Here's the drawing with two shaded views (mm, measured from the low corner). I have some questions. A direction names the side the tool comes from. Round coordinates to 2 decimals unless told otherwise and drop trailing zeros. Loops run counter-clockwise (first coordinate to the right, second up) from the corner with the lowest first, then second, coordinate; pieces in that order, holes last. Notation, with made-up numbers: M 89.25,65 L 141.25,65 A18 ccw 141.25,82 Z; hole C -29,81.25 d3. An arc over 180 degrees is marked long. Answer as CSV lines item,"result".
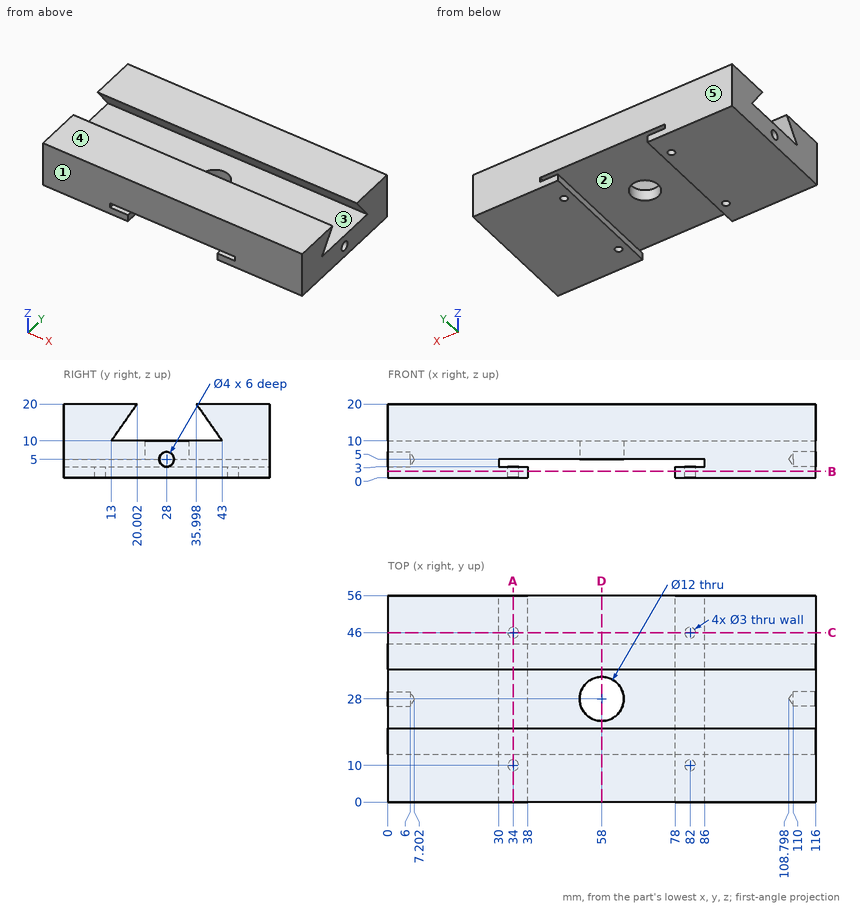
1. I want a section at D-D, the plane x = 58. Please give me the cut outline in (y, z), and give its area (3 significant figures).
Evaluation:
outline,"M 0,5 L 22,5 L 22,10 L 13,10 L 20,20 L 0,20 Z; M 34,5 L 56,5 L 56,20 L 36,20 L 43,10 L 34,10 Z"
area,"550 mm²"
2. We'd pull the mould along Y, two halves only. Please class the marked faces 3, 4 and 5: pulls with the +Y half, pulls with the -Y half, needs draft (parallel to the pull), parting line crosses it, or undercut.
Evaluation:
face 3,"undercut"
face 4,"needs draft"
face 5,"pulls with the +Y half"
3. I want a section at B-B, the plane z = 1.75. Please give me the cut outline in (x, y), and give its area (3 significant figures).
Evaluation:
outline,"M 0,0 L 38,0 L 38,56 L 0,56 Z; M 78,0 L 116,0 L 116,56 L 78,56 Z; hole C 34,10 d3; hole C 34,46 d3; hole C 82,10 d3; hole C 82,46 d3"
area,"4,230 mm²"
4. I want a section at A-A, the plane x = 34. Please give me the cut outline in (y, z), and give its area (3 significant figures).
Evaluation:
outline,"M 0,0 L 8.5,0 L 8.5,3 L 0,3 Z; M 0,5 L 56,5 L 56,20 L 36,20 L 43,10 L 13,10 L 20,20 L 0,20 Z; M 11.5,0 L 44.5,0 L 44.5,3 L 11.5,3 Z; M 47.5,0 L 56,0 L 56,3 L 47.5,3 Z"
area,"760 mm²"
5. I want a section at C-C, the plane y = 46. Please give me the cut outline in (x, z), and give its area (3 significant figures).
Evaluation:
outline,"M 0,0 L 32.5,0 L 32.5,3 L 30,3 L 30,5 L 86,5 L 86,3 L 83.5,3 L 83.5,0 L 116,0 L 116,20 L 0,20 Z; M 35.5,0 L 38,0 L 38,3 L 35.5,3 Z; M 78,0 L 80.5,0 L 80.5,3 L 78,3 Z"
area,"2,070 mm²"
6. For P1, Ø2.5, axis at y = 28, z = 5, coming from the +X side; P2, Ø1, axis at y = 27, z = 4, coming from the +X side; P3, Ø1.8, axis at x = 34, y = 46, coming from the -Z side; P4, Ø11, axis at x = 58, y = 28, coming from the +Z side, each with a flat end and sliding along its axis, tell me the tip position at first contact or that it passes through.
Evaluation:
P1,"stops at x = 109.55"
P2,"stops at x = 109.95"
P3,"stops at z = 5"
P4,"passes through"
7. Which directions (+Z, -Z, +X, -X, +Y, -Y) give clear straight access to the entire face, cutting with the end or side of a thin tool? Please do the marked faces 1 and 2.
Evaluation:
face 1,"+Z, -Z, +X, -X, -Y"
face 2,"+Y, -Y"
8. If I drill on line 1 (Y direction, x = 34, z = 1.3); line 2 (X direction, y = 45.5, z = 1.25) (1 decimal); line 3 (Z direction, x = 85.5, y = 16) (1 decimal), over which ranges is the centre line in solid material (lowest first)? Write a range as [from, to].
Evaluation:
line 1,"y = [0, 8.5], [11.5, 44.5], [47.5, 56]"
line 2,"x = [0, 32.6], [35.4, 38], [78, 80.6], [83.4, 116]"
line 3,"z = [0, 3], [5, 10], [14.3, 20]"
